For this review, take the finished solid that the model builds, in its own axes (mm). Face numbers are marked on the shaded views. A direction names the side the tool comes from. Give positions to 0.01 mm unless a question says otherwise; leave off trailing zeros. Write each loop counter-clockwise with the first axis right and the second up, starting at its lowest first coordinate (ties: lowest second). Pieces come first, ordered by that corner, then holes. Notation, with made-up numbers: M 53,13.5 L 85,13.5 A19 ccw 85,35.5 Z; hole C 31,-22 d9. An arc over 180 degrees is marked long. One line per item, written item: value. Start each with the question number.
Item 1: Clearance check with flat-ended pins moving along their axes: pin 1 Ø1.9 at (x, y) = (0, -11) entering from -Z; pin 2 Ø1.1 at (x, y) = (26, 0) entering from -Z; pin 3 Ø5 at (x, y) = (6, -4.5) entering from +Z; pin 4 Ø12 at (x, z) = (-7.5, 12) entering from +Y. State where each tip first meets the part, or that it passes through.
Item 2: To check wall thickness, follow probe 1 along X at (y, z) = (-5, 27); probe 2 along X at (y, z) = (3.25, -3); probe 3 along Y at (x, z) = (9.5, 28). State the ranges of each line that lie inside material, in increasing order.
Item 3: Consider section A-A, the plane x = 22.5. Write out the cut boundary in (y, z), and give its area (3 significant figures).
Item 4: Mouldability with a two-part tool opening along X and no side actions: class the marked faces 1, 2 and 3 as released by +X, released by -X, zero draft, split by the parting line, or undercut.
Item 5: Tool access review of the marked faces 4, 5 and 6: name each direction out of +Z, -Z, +X, -X, +Y, -Y from which nothing blocks a thin tool from reaching the whole face with its end or side.
Item 6: Consider section B-B, the plane z = 10.5. Write out the cut boundary in (x, y), and give its area (3 significant figures).
```python
from build123d import *

# Parameters (mm, degrees)
BODY_DEPTH                       = 32
BODY_DEPTH_BACK                  = 15
PIVOT_START                      = 25
PIVOT_PIN_R_SKETCH_R             = 4
PIVOT_PIN_R_DEPTH                = 4.25
OUTSIDE_SHAPE_CUT_OUT_DEPTH      = 46.245165488
OUTSIDE_SHAPE_CUT_OUT_DEPTH_BACK = 46.245165488
OUTSIDE_SHAPE_CUT_OUT_SKETCH_W   = 49
OUTSIDE_SHAPE_CUT_OUT_SKETCH_H   = 25.5
OUTSIDE_START                    = 27.3
OUTSIDE_SHAPE_CUT_OUT_SKETCH_R_W = 24
OUTSIDE_SHAPE_CUT_OUT_SKETCH_R_H = 24
OUTSIDE_SHAPE_CUT_OUT_SKETCH_R_R = 4
OUTSIDE_SHAPE_CUT_OUT_R_DEPTH    = 18.945165488
INSIDE_START                     = 25
INSIDE_SHAPE_CUT_OUT_DEPTH       = 50
LIGHTENING_START                 = 1.25
LIGHTENING_2_SKETCH_W            = 55.1
LIGHTENING_2_SKETCH_H            = 5.5
LIGHTENING_2_DEPTH               = 44.995165488
F_3_START                        = -11.75
F_3_M5_SLOTS_DEPTH               = 3.5


with BuildPart() as part:
    # Profile Sketch → Body (new, two sides: drawn at the far end of the back side and taken through both)
    with BuildSketch(Plane.XY.offset(-BODY_DEPTH_BACK)):
        Polygon((-29.75, -11.75), (29.75, -11.75), (29.75, 11.75), (25, 11.75), (25, -8.25), (-25, -8.25), (-25, 11.75), (-29.75, 11.75), align=None)
    extrude(amount=BODY_DEPTH + BODY_DEPTH_BACK)

    # Pivot Pin R Sketch → Pivot Pin R (add)
    with BuildSketch(Plane(origin=(0, 0, 0), x_dir=(0, 0, -1), z_dir=(1, 0, 0)).offset(PIVOT_START)):
        Circle(PIVOT_PIN_R_SKETCH_R)
    pivot_pin_r = extrude(amount=PIVOT_PIN_R_DEPTH)

    # Pivot Pin L: Pivot Pin R across plane
    add(pivot_pin_r.mirror(Plane(origin=(0, 0, 0), x_dir=(0, 0, 1), z_dir=(1, 0, 0))))

    # Outside Shape Cut Out Sketch → Outside Shape Cut Out (cut, two sides: drawn at the far end of the back side and taken through both)
    with BuildSketch(Plane(origin=(0, 0, 0), x_dir=(0, 0, -1), z_dir=(1, 0, 0)).offset(-OUTSIDE_SHAPE_CUT_OUT_DEPTH_BACK)):
        with Locations((-9.5, -1)):
            Rectangle(OUTSIDE_SHAPE_CUT_OUT_SKETCH_W, OUTSIDE_SHAPE_CUT_OUT_SKETCH_H)
        with BuildLine():
            Line((-27.879626464, 3.486362585), (-9.617692031, 6.75))
            ThreePointArc((-9.617692031, 6.75), (-6.204756601, 9.978150907), (-1.8, 11.611309142))
            Line((-1.8, 11.611309142), (-1.3, 7.9))
            Line((-1.3, 7.9), (1.3, 7.9))
            Line((1.3, 7.9), (1.8, 11.611309142))
            ThreePointArc((1.8, 11.611309142), (8.308504679, 8.308504679), (11.611309142, 1.8))
            Line((11.611309142, 1.8), (7.9, 1.3))
            Line((7.9, 1.3), (7.9, -1.3))
            Line((7.9, -1.3), (11.611309142, -1.8))
            ThreePointArc((11.611309142, -1.8), (7.645668708, -8.922233465), (0, -11.75))
            Line((0, -11.75), (-32, -11.75))
            Line((-32, -11.75), (-32, -1.435655018))
            ThreePointArc((-32, -1.435655018), (-30.833936118, 1.773851772), (-27.879626464, 3.486362585))
        make_face(mode=Mode.SUBTRACT)
    extrude(amount=OUTSIDE_SHAPE_CUT_OUT_DEPTH + OUTSIDE_SHAPE_CUT_OUT_DEPTH_BACK, mode=Mode.SUBTRACT)

    # Outside Shape Cut Out Sketch R → Outside Shape Cut Out R (cut, through all)
    with BuildSketch(Plane(origin=(0, 0, 0), x_dir=(0, 0, -1), z_dir=(1, 0, 0)).offset(OUTSIDE_START)):
        Rectangle(OUTSIDE_SHAPE_CUT_OUT_SKETCH_R_W, OUTSIDE_SHAPE_CUT_OUT_SKETCH_R_H)
        Circle(OUTSIDE_SHAPE_CUT_OUT_SKETCH_R_R, mode=Mode.SUBTRACT)
    outside_shape_cut_out_r = extrude(amount=OUTSIDE_SHAPE_CUT_OUT_R_DEPTH, mode=Mode.SUBTRACT)

    # Outside Shape Cut Out L: Outside Shape Cut Out R across plane
    add(outside_shape_cut_out_r.mirror(Plane(origin=(0, 0, 0), x_dir=(0, 0, 1), z_dir=(1, 0, 0))), mode=Mode.SUBTRACT)

    # Inside Shape Cut Out Sketch → Inside Shape Cut Out (cut)
    with BuildSketch(Plane(origin=(0, 0, 0), x_dir=(0, 0, -1), z_dir=(1, 0, 0)).offset(INSIDE_START)):
        Polygon((-29, -9.75), (-29, -11.75), (-32, -11.75), (-32, -10.75), (-30.5, -10.75), (-30.5, -9.75), align=None)
        Polygon((-9.5, -8.25), (-5, -10.75), (-5, -11.75), (8.366600265, -11.75), (8.366600265, -8.25), align=None)
    extrude(amount=-INSIDE_SHAPE_CUT_OUT_DEPTH, mode=Mode.SUBTRACT)

    # Lightening 2 Sketch → Lightening 2 (cut, through all)
    with BuildSketch(Plane(origin=(0, 0, 0), x_dir=(1, 0, 0), z_dir=(0, 1, 0)).offset(LIGHTENING_START)):
        with Locations((0, -18.25)):
            Rectangle(LIGHTENING_2_SKETCH_W, LIGHTENING_2_SKETCH_H)
    extrude(amount=LIGHTENING_2_DEPTH, mode=Mode.SUBTRACT)

    # 3 M5 Slots: read off the stored shape, not the designer's step
    # 3 M5 Slots outline → 3 M5 Slots (cut)
    with BuildSketch(Plane(origin=(0, 0, 0), x_dir=(1, 0, 0), z_dir=(0, 1, 0)).offset(F_3_START)):
        with BuildLine():
            Line((-0.85, -20.65), (0.85, -20.65))
            ThreePointArc((0.85, -20.65), (3.5, -18), (0.85, -15.35))
            Line((0.85, -15.35), (-0.85, -15.35))
            ThreePointArc((-0.85, -15.35), (-3.5, -18), (-0.85, -20.65))
        make_face()
        with BuildLine():
            Line((13.15, -27.65), (14.85, -27.65))
            ThreePointArc((14.85, -27.65), (17.5, -25), (14.85, -22.35))
            Line((14.85, -22.35), (13.15, -22.35))
            ThreePointArc((13.15, -22.35), (10.5, -25), (13.15, -27.65))
        make_face()
        with BuildLine():
            ThreePointArc((-13.15, -27.65), (-10.5, -25), (-13.15, -22.35))
            Line((-13.15, -22.35), (-14.85, -22.35))
            ThreePointArc((-14.85, -22.35), (-17.5, -25), (-14.85, -27.65))
            Line((-14.85, -27.65), (-13.15, -27.65))
        make_face()
    extrude(amount=F_3_M5_SLOTS_DEPTH, mode=Mode.SUBTRACT)

    # 3 M5 Slots 2: loft between two sections, ruled curve by curve
    f_3_m5_slots_2_from = [
        Edge.make_three_point_arc((0.85, -9.6, 20.65), (2.72383297, -9.6, 19.87383297), (3.5, -9.6, 18)),
        Edge.make_three_point_arc((3.5, -9.6, 18), (2.72383297, -9.6, 16.12616703), (0.85, -9.6, 15.35)),
        Edge.make_three_point_arc((-0.85, -9.6, 15.35), (-2.72383297, -9.6, 16.12616703), (-3.5, -9.6, 18)),
        Edge.make_three_point_arc((-3.5, -9.6, 18), (-2.72383297, -9.6, 19.87383297), (-0.85, -9.6, 20.65)),
        Edge.make_line((0.85, -9.6, 15.35), (-0.85, -9.6, 15.35)),
        Edge.make_line((0.85, -9.6, 20.65), (-0.85, -9.6, 20.65)),
    ]
    f_3_m5_slots_2_to = [
        Edge.make_three_point_arc((0.85, -8.25, 22), (3.678427125, -8.25, 20.828427125), (4.85, -8.25, 18)),
        Edge.make_three_point_arc((4.85, -8.25, 18), (3.678427125, -8.25, 15.171572875), (0.85, -8.25, 14)),
        Edge.make_three_point_arc((-0.85, -8.25, 14), (-3.678427125, -8.25, 15.171572875), (-4.85, -8.25, 18)),
        Edge.make_three_point_arc((-4.85, -8.25, 18), (-3.678427125, -8.25, 20.828427125), (-0.85, -8.25, 22)),
        Edge.make_line((0.85, -8.25, 14), (-0.85, -8.25, 14)),
        Edge.make_line((0.85, -8.25, 22), (-0.85, -8.25, 22)),
    ]
    f_3_m5_slots_2 = Solid(Shell([*[Face.make_surface_from_curves(f_3_m5_slots_2_from[k], f_3_m5_slots_2_to[k]) for k in range(6)], Face(Wire(f_3_m5_slots_2_from)), Face(Wire(f_3_m5_slots_2_to))]))
    add(f_3_m5_slots_2, mode=Mode.SUBTRACT)

    # 3 M5 Slots 3: loft between two sections, ruled curve by curve
    f_3_m5_slots_3_from = [
        Edge.make_three_point_arc((14.85, -9.6, 27.65), (16.72383297, -9.6, 26.87383297), (17.5, -9.6, 25)),
        Edge.make_three_point_arc((17.5, -9.6, 25), (16.72383297, -9.6, 23.12616703), (14.85, -9.6, 22.35)),
        Edge.make_three_point_arc((13.15, -9.6, 22.35), (11.27616703, -9.6, 23.12616703), (10.5, -9.6, 25)),
        Edge.make_three_point_arc((10.5, -9.6, 25), (11.27616703, -9.6, 26.87383297), (13.15, -9.6, 27.65)),
        Edge.make_line((14.85, -9.6, 22.35), (13.15, -9.6, 22.35)),
        Edge.make_line((14.85, -9.6, 27.65), (13.15, -9.6, 27.65)),
    ]
    f_3_m5_slots_3_to = [
        Edge.make_three_point_arc((14.85, -8.25, 29), (17.678427125, -8.25, 27.828427125), (18.85, -8.25, 25)),
        Edge.make_three_point_arc((18.85, -8.25, 25), (17.678427125, -8.25, 22.171572875), (14.85, -8.25, 21)),
        Edge.make_three_point_arc((13.15, -8.25, 21), (10.321572875, -8.25, 22.171572875), (9.15, -8.25, 25)),
        Edge.make_three_point_arc((9.15, -8.25, 25), (10.321572875, -8.25, 27.828427125), (13.15, -8.25, 29)),
        Edge.make_line((14.85, -8.25, 21), (13.15, -8.25, 21)),
        Edge.make_line((14.85, -8.25, 29), (13.15, -8.25, 29)),
    ]
    f_3_m5_slots_3 = Solid(Shell([*[Face.make_surface_from_curves(f_3_m5_slots_3_from[k], f_3_m5_slots_3_to[k]) for k in range(6)], Face(Wire(f_3_m5_slots_3_from)), Face(Wire(f_3_m5_slots_3_to))]))
    add(f_3_m5_slots_3, mode=Mode.SUBTRACT)

    # 3 M5 Slots 4: loft between two sections, ruled curve by curve
    f_3_m5_slots_4_from = [
        Edge.make_three_point_arc((-13.15, -9.6, 27.65), (-11.27616703, -9.6, 26.87383297), (-10.5, -9.6, 25)),
        Edge.make_three_point_arc((-10.5, -9.6, 25), (-11.27616703, -9.6, 23.12616703), (-13.15, -9.6, 22.35)),
        Edge.make_three_point_arc((-14.85, -9.6, 22.35), (-16.72383297, -9.6, 23.12616703), (-17.5, -9.6, 25)),
        Edge.make_three_point_arc((-17.5, -9.6, 25), (-16.72383297, -9.6, 26.87383297), (-14.85, -9.6, 27.65)),
        Edge.make_line((-13.15, -9.6, 22.35), (-14.85, -9.6, 22.35)),
        Edge.make_line((-13.15, -9.6, 27.65), (-14.85, -9.6, 27.65)),
    ]
    f_3_m5_slots_4_to = [
        Edge.make_three_point_arc((-13.15, -8.25, 29), (-10.321572875, -8.25, 27.828427125), (-9.15, -8.25, 25)),
        Edge.make_three_point_arc((-9.15, -8.25, 25), (-10.321572875, -8.25, 22.171572875), (-13.15, -8.25, 21)),
        Edge.make_three_point_arc((-14.85, -8.25, 21), (-17.678427125, -8.25, 22.171572875), (-18.85, -8.25, 25)),
        Edge.make_three_point_arc((-18.85, -8.25, 25), (-17.678427125, -8.25, 27.828427125), (-14.85, -8.25, 29)),
        Edge.make_line((-13.15, -8.25, 21), (-14.85, -8.25, 21)),
        Edge.make_line((-13.15, -8.25, 29), (-14.85, -8.25, 29)),
    ]
    f_3_m5_slots_4 = Solid(Shell([*[Face.make_surface_from_curves(f_3_m5_slots_4_from[k], f_3_m5_slots_4_to[k]) for k in range(6)], Face(Wire(f_3_m5_slots_4_from)), Face(Wire(f_3_m5_slots_4_to))]))
    add(f_3_m5_slots_4, mode=Mode.SUBTRACT)


solid = part.part
```
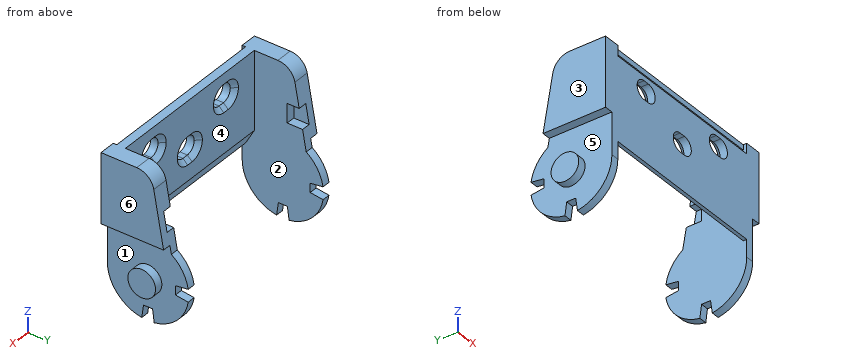
Model answer:
1. pin 1: stops at z = 5
1. pin 2: stops at z = -7.9
1. pin 3: passes through
1. pin 4: stops at y = -8.25
2. probe 1: x = -29.75 to -25, 25 to 29.75
2. probe 2: x = -27.3 to -25, 25 to 27.3
2. probe 3: y = -11.75 to -8.25
3. outline: M -11.75,5 L -10.75,5 L -8.25,9.5 L -8.25,32 L -10.75,32 L -10.75,30.5 L -9.75,30.5 L -9.75,29 L -11.75,29 Z
3. area: 84.4 mm2
4. face 1: released by +X
4. face 2: undercut
4. face 3: released by -X
5. face 4: +Z, -Z, +Y
5. face 5: -X
5. face 6: +Z, -Z, +X, +Y, -Y
6. outline: M -27.3,-11.75 L 27.3,-11.75 L 27.3,6.59 L 25,6.59 L 25,-8.25 L -25,-8.25 L -25,6.59 L -27.3,6.59 Z
6. area: 259 mm2
